Check sheet for the modelled part. Datum: model origin and axes. Units: mm. Face numbers are marked on the shaded views. Give positions to 0.01 mm unless a question says otherwise; leave off trailing zeros. Write each loop counter-clockwise with the first axis right and the second up, starting at its lowest first coordinate (ties: lowest second). Pieces come first, ordered by that corner, then holes. Notation, with made-up numbers: (47, -26) -> (60, -26) arc R20 cw to (60, -22) -> close; hole circle Ø4 at (61.5, 86.25). An arc over 180 degrees is marked (long way). Answer as a JSON object with one key per item and string values.
from build123d import *

# Parameters (mm, degrees)
SKETCH_1_R               = 48.25
SKETCH_1_R_2             = 38
EXTRUDE_1_DEPTH          = 10
SKETCH_2_R               = 38
SKETCH_2_R_2             = 36
EXTRUDE_2_DEPTH          = 2
SKETCH_3_R               = 1.775
CUT_EXTRUDE_1_DEPTH      = 1
CUT_EXTRUDE_1_DEPTH_BACK = 11
SKETCH_4_R               = 2
EXTRUDE_3_DEPTH          = 10
SKETCH_5_R               = 1.775
CUT_EXTRUDE_2_DEPTH      = 10


with BuildPart() as part:
    # 草图1 → 凸台-拉伸1 (new body)
    with BuildSketch(Plane(origin=(0, 0, 0), x_dir=(1, 0, 0), z_dir=(0, 1, 0))):
        Circle(SKETCH_1_R)
        Circle(SKETCH_1_R_2, mode=Mode.SUBTRACT)
    extrude(amount=EXTRUDE_1_DEPTH)

    # 草图2 → 凸台-拉伸2 (add)
    with BuildSketch(Plane(origin=(0, 10, 0), x_dir=(1, 0, 0), z_dir=(0, 1, 0))):
        Circle(SKETCH_2_R)
        Circle(SKETCH_2_R_2, mode=Mode.SUBTRACT)
    extrude(amount=-EXTRUDE_2_DEPTH)

    # 草图3 → 切除-拉伸1 (cut, two sides)
    with BuildSketch(Plane.XZ) as cut_extrude_1_sk:
        with Locations((0, 44.5)):
            Circle(SKETCH_3_R)
        with Locations((31.466251763, 31.466251763)):
            Circle(SKETCH_3_R)
        with Locations((44.5, 0)):
            Circle(SKETCH_3_R)
        with Locations((31.466251763, -31.466251763)):
            Circle(SKETCH_3_R)
        with Locations((0, -44.5)):
            Circle(SKETCH_3_R)
        with Locations((-31.466251763, -31.466251763)):
            Circle(SKETCH_3_R)
        with Locations((-44.5, 0)):
            Circle(SKETCH_3_R)
        with Locations((-31.466251763, 31.466251763)):
            Circle(SKETCH_3_R)
    extrude(amount=CUT_EXTRUDE_1_DEPTH, mode=Mode.SUBTRACT)
    extrude(cut_extrude_1_sk.sketch, amount=-CUT_EXTRUDE_1_DEPTH_BACK, mode=Mode.SUBTRACT)

    # 草图4 → 凸台-拉伸3 (add)
    with BuildSketch(Plane(origin=(0, 10, 0), x_dir=(1, 0, 0), z_dir=(0, 1, 0))):
        with Locations((0, -44.5)):
            Circle(SKETCH_4_R)
        with Locations((0, 44.5)):
            Circle(SKETCH_4_R)
    extrude(amount=-EXTRUDE_3_DEPTH)

    # 草图5 → 切除-拉伸2 (cut)
    with BuildSketch(Plane(origin=(0, 10, 0), x_dir=(1, 0, 0), z_dir=(0, 1, 0))):
        with Locations((5.5258e-05, -42.50007959)):
            Circle(SKETCH_5_R)
        with Locations((2.4326e-05, 42.499999999)):
            Circle(SKETCH_5_R)
    extrude(amount=-CUT_EXTRUDE_2_DEPTH, mode=Mode.SUBTRACT)


solid = part.part
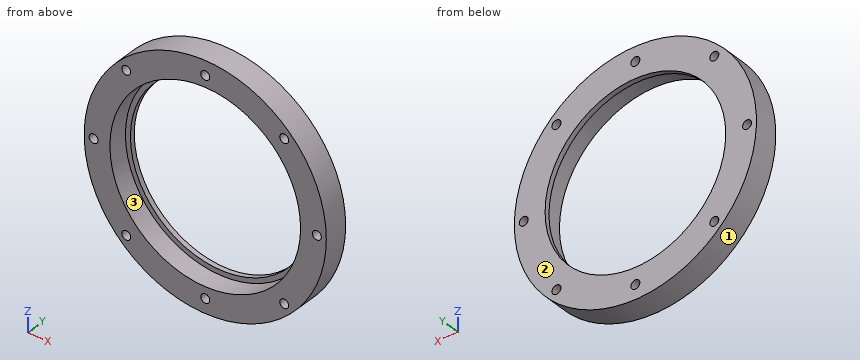
1. Mould release check, pull along X, two halves, no side actions. Record for the marked faces 1, 2 and 3: released by +X, released by -X, zero draft, split by the parting line, or undercut.
Determined:
{"face 1": "split by the parting line", "face 2": "zero draft", "face 3": "undercut"}
2. Go/stop test with flat-tipped pins: P1, Ø1, axis at x = -33, y = 7, coming from the -Z side; P2, Ø3, axis at x = -31.47, z = 31.47, coming from the -Y side; P3, Ø1.5, axis at y = 2, z = 35.5, coming from the +X side; P4, Ø1.5, axis at x = 5, y = 4, coming from the +Z side. Record where each tip stops, or that it passes through.
Determined:
{"P1": "z = -35.66", "P2": "through", "P3": "x = 33.47", "P4": "z = 48.06"}
3. Sectioned sample at D-D, the plane z = 14. Enter the section's corners in (x, y), plus the area to 3 significant figures.
Determined:
{"outline": "(-46.17, 0) -> (-35.33, 0) -> (-35.33, 8) -> (-33.17, 8) -> (-33.17, 10) -> (-46.17, 10) -> close; (33.17, 8) -> (35.33, 8) -> (35.33, 0) -> (46.17, 0) -> (46.17, 10) -> (33.17, 10) -> close", "area": "226 mm^2"}
4. Sectioned sample at B-B, the plane x = 0. Enter the section's corners in (y, z) (3 decimals).
Determined:
{"outline": "(0, -48.25) -> (10, -48.25) -> (10, -44.275) -> (0, -44.275) -> close; (0, -40.725) -> (10, -40.725) -> (10, -36) -> (8, -36) -> (8, -38) -> (0, -38) -> close; (0, 38) -> (8, 38) -> (8, 36) -> (10, 36) -> (10, 40.725) -> (0, 40.725) -> close; (0, 44.275) -> (10, 44.275) -> (10, 48.25) -> (0, 48.25) -> close"}
5. Sectioned sample at A-A, the plane z = 0. Enter the section's corners in (x, y) (3 decimals), plus the area to 3 significant figures.
Determined:
{"outline": "(-48.25, 0) -> (-46.275, 0) -> (-46.275, 10) -> (-48.25, 10) -> close; (-42.725, 0) -> (-38, 0) -> (-38, 8) -> (-36, 8) -> (-36, 10) -> (-42.725, 10) -> close; (36, 8) -> (38, 8) -> (38, 0) -> (42.725, 0) -> (42.725, 10) -> (36, 10) -> close; (46.275, 0) -> (48.25, 0) -> (48.25, 10) -> (46.275, 10) -> close", "area": "142 mm^2"}
6. Scan lines: L1, parallel to Z at x = -12, y = 2.5; L2, parallel to Z at x = -23, y = 1; L3, parallel to X at y = 9, z = 5. Record each from-to range of solid material in increasing order. Write a range as [from, to].
Determined:
{"L1": "[-46.73, -36.06], [36.06, 46.73]", "L2": "[-42.42, -30.25], [30.25, 42.42]", "L3": "[-47.99, -35.65], [35.65, 47.99]"}
7. Sectioned sample at C-C, the plane x = 11. Enter the section's corners in (y, z), plus the area to 3 significant figures.
Determined:
{"outline": "(0, -46.98) -> (10, -46.98) -> (10, -34.28) -> (8, -34.28) -> (8, -36.37) -> (0, -36.37) -> close; (0, 36.37) -> (8, 36.37) -> (8, 34.28) -> (10, 34.28) -> (10, 46.98) -> (0, 46.98) -> close", "area": "221 mm^2"}
